Model file for the job. Use its own axes, mm. Face numbers are marked on the shaded views. A direction names the side the tool comes from. Round coordinates to 2 decimals unless told otherwise and drop trailing zeros. Loops run counter-clockwise (first coordinate to the right, second up) from the corner with the lowest first, then second, coordinate; pieces in that order, holes last. Notation, with made-up numbers: M 32,79.25 L 87,79.25 A30 cw 87,107.25 Z; hole C 80,4.5 d10. An arc over 180 degrees is marked long. Answer in a Markdown table with one row per item.
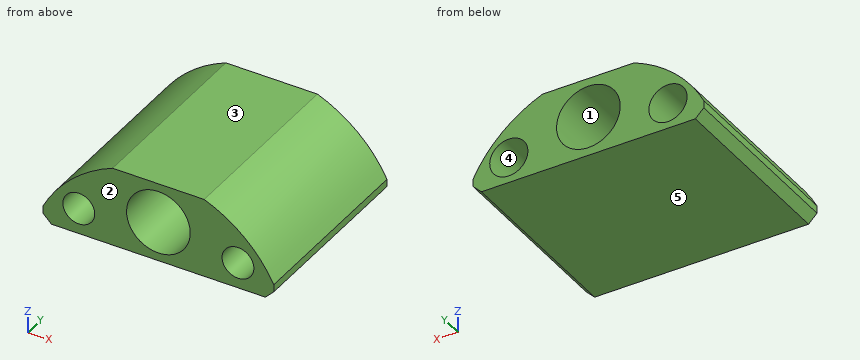
from build123d import *

# Parameters (mm, degrees)
BOSS_EXTRUDE1_DEPTH = 47
SKETCH2_R           = 4
SKETCH2_R_2         = 8
CUT_EXTRUDE1_DEPTH  = 59.736700622
SKETCH3_R           = 4.8
CUT_EXTRUDE2_DEPTH  = 37.5


with BuildPart() as part:
    # Sketch1 → Boss-Extrude1 (new body)
    with BuildSketch(Plane(origin=(0, 0, 0), x_dir=(1, 0, 0), z_dir=(0, 1, 0))):
        with BuildLine():
            Line((-26.878679656, 0), (26.878679656, 0))
            Line((26.878679656, 0), (29, -2.121320344))
            Line((29, -2.121320344), (29, -4))
            ThreePointArc((29, -4), (21.712972029, -13.600125657), (11.5, -20))
            Line((11.5, -20), (-11.5, -20))
            ThreePointArc((-11.5, -20), (-21.712972029, -13.600125657), (-29, -4))
            Line((-29, -4), (-29, -2.121320344))
            Line((-29, -2.121320344), (-26.878679656, 0))
        make_face()
    extrude(amount=-BOSS_EXTRUDE1_DEPTH)

    # Sketch2 → Cut-Extrude1 (cut, through all)
    with BuildSketch(Plane(origin=(0, 0, 0), x_dir=(1, 0, 0), z_dir=(0, 1, 0))):
        with Locations(Location((-20, -6.5, 0), (0, 0, 270))):
            Circle(SKETCH2_R)
        with Locations(Location((0, -10, 0), (0, 0, 270))):
            Circle(SKETCH2_R_2)
        with Locations(Location((20, -6.5, 0), (0, 0, 270))):
            Circle(SKETCH2_R)
    extrude(amount=-CUT_EXTRUDE1_DEPTH, mode=Mode.SUBTRACT)

    # Sketch3 → Cut-Extrude2 (cut)
    with BuildSketch(Plane(origin=(0, 0, 0), x_dir=(1, 0, 0), z_dir=(0, 1, 0))):
        with Locations(Location((-20, -6.5, 0), (0, 0, 270))):
            Circle(SKETCH3_R)
        with Locations(Location((20, -6.5, 0), (0, 0, 270))):
            Circle(SKETCH3_R)
    extrude(amount=-CUT_EXTRUDE2_DEPTH, mode=Mode.SUBTRACT)


solid = part.part
1. Pin check, flat tips, straight feed: pin 1 (2 mm diameter, centred on y = -6.5, z = 7, fed in from -X); pin 2 (6 mm diameter, centred on x = 19, y = -29.5, fed in from +Z). Stop position of each tip, or through.
Verdict:
| item | result |
|---|---|
| pin 1 | stops at x = -27.9 |
| pin 2 | stops at z = 17.81 |
2. Mould opens along Z. For the marked faces 1, 2 and 3 say: +Z half, -Z half, draft (parallel to the pull), parting line (faces both ways), or undercut.
Verdict:
| item | result |
|---|---|
| face 1 | undercut |
| face 2 | draft |
| face 3 | +Z half |
3. Saw through at B-B (x = 0). Write the cut outline in (y, z), and give its area (3 significant figures).
Verdict:
| item | result |
|---|---|
| outline | M -47,0 L 0,0 L 0,2 L -47,2 Z; M -47,18 L 0,18 L 0,20 L -47,20 Z |
| area | 188 mm² |
4. Wall check: probe 1 along X at (y, z) = (-28, 6.5); probe 2 along X at (y, z) = (-15, 10); probe 3 along Z at (x, y) = (-21.5, -31). Give the ranges that are in metal, low to high.
Verdict:
| item | result |
|---|---|
| probe 1 | x = -27.6 to -24.8, -15.2 to -7.19, 7.19 to 15.2, 24.8 to 27.6 |
| probe 2 | x = -25.11 to -23.28, -16.72 to -8, 8 to 16.72, 23.28 to 25.11 |
| probe 3 | z = 0 to 1.94, 11.06 to 13.79 |
5. Tool access for the marked faces 4 and 5: list every direction of +Z, -Z, +X, -X, +Y, -Y with a clear straight run to the whole face (end or side of a thin tool).
Verdict:
| item | result |
|---|---|
| face 4 | +Y |
| face 5 | -Z, +X, -X, +Y, -Y |
6. Saw through at C-C (y = -36). Write the cut outline in (x, z), and give its area (3 significant figures).
Verdict:
| item | result |
|---|---|
| outline | M -29,2.12 L -26.88,0 L 26.88,0 L 29,2.12 L 29,4 A33.5 ccw 11.5,20 L -11.5,20 A33.5 ccw -29,4 Z; hole C -20,6.5 d9.6; hole C 0,10 d16; hole C 20,6.5 d9.6 |
| area | 599 mm² |
7. Saw through at A-A (z = 6.5). Write the cut outline in (x, y), and give its area (3 significant figures).
Verdict:
| item | result |
|---|---|
| outline | M -27.6,-47 L -24,-47 L -24,-37.5 L -24.8,-37.5 L -24.8,0 L -27.6,0 Z; M -16,-47 L -7.19,-47 L -7.19,0 L -15.2,0 L -15.2,-37.5 L -16,-37.5 Z; M 7.19,-47 L 16,-47 L 16,-37.5 L 15.2,-37.5 L 15.2,0 L 7.19,0 Z; M 24,-47 L 27.6,-47 L 27.6,0 L 24.8,0 L 24.8,-37.5 L 24,-37.5 Z |
| area | 1,050 mm² |
8. Saw through at D-D (x = -20). Write the cut outline in (y, z), and give its area (3 significant figures).
Verdict:
| item | result |
|---|---|
| outline | M -47,0 L 0,0 L 0,1.7 L -37.5,1.7 L -37.5,2.5 L -47,2.5 Z; M -47,10.5 L -37.5,10.5 L -37.5,11.3 L 0,11.3 L 0,15.06 L -47,15.06 Z |
| area | 272 mm² |
